from build123d import *

# Parameters (mm, degrees)
F0_W     = 20.1
F0_H     = 40.9
F0_W_2   = 15.1
F0_H_2   = 35.9
F1_DEPTH = 22
F2_DEPTH = 19.5
F4_R     = 1.695
F5_DEPTH = 25
F7_W     = 3.375
F7_H     = 4.11
F8_DEPTH = 25


with BuildPart() as f1:
    # F0 (on Top) → F1 (new body)
    with BuildSketch(Plane.XY):
        with Locations((7.55, 24.2)):
            Rectangle(F0_W, F0_H)
        with Locations((7.55, 24.2)):
            Rectangle(F0_W_2, F0_H_2, mode=Mode.SUBTRACT)
        with Locations((7.55, 24.2)):
            Rectangle(F0_W_2, F0_H_2)
    extrude(amount=F1_DEPTH)

    # F0 (on Top) → F2 (cut)
    with BuildSketch(Plane.XY):
        with Locations((7.55, 24.2)):
            Rectangle(F0_W_2, F0_H_2)
    extrude(amount=F2_DEPTH, mode=Mode.SUBTRACT)

    # F4 (on offset) → F5 (cut)
    with BuildSketch(Plane.XY.offset(22)):
        with Locations((4.5, 37.65)):
            Circle(F4_R)
        with Locations((10.6, 37.65)):
            Circle(F4_R)
        with Locations((4.5, 10.75)):
            Circle(F4_R)
        with Locations((10.6, 10.75)):
            Circle(F4_R)
    extrude(amount=-F5_DEPTH, mode=Mode.SUBTRACT)

    # F7 (on offset) → F8 (cut)
    with BuildSketch(Plane(origin=(0, 44.65, 0), x_dir=(-1, 0, 0), z_dir=(0, 1, 0))):
        with Locations((-5.8625, 15.2)):
            Rectangle(F7_W, F7_H)
        with Locations((-9.2375, 15.2)):
            Rectangle(F7_W, F7_H)
    extrude(amount=-F8_DEPTH, mode=Mode.SUBTRACT)


solid = f1.part
Part model, mm, in its own coordinate system. A direction names the side the tool comes from. Coordinates: 2 decimals unless noted, no trailing zeros. Loops run counter-clockwise (first coordinate to the right, second up) from the corner with the lowest first, then second, coordinate; pieces in that order, holes last. Notation, with made-up numbers: M 12.5,25.25 L 27.5,25.25 A17 cw 27.5,54.25 Z; hole C 39.25,29.5 d3. An arc over 180 degrees is marked long. Use a Markdown table: item, result. Add a question column.
Q1. Which spindle directions (+Z, -Z, +X, -X, +Y, -Y) get a long thin tool onto all of the face, cutting with end or side? Do faces 5 (the flat face through (15.1, 24, 10)), 6 (the flat face through (8, 43, 17.255)), 7 (the flat face through (-1, 23, 0)). Say none if no direction does.
Q2. Cut at A-A (y = 10.75). Write the cut outline in (x, z) (3 decimals), and give its area (3 significant figures).
Q3. Pin check, flat tips, straight feed: P1, Ø4, axis at x = 13, y = 25.5, coming from the -Z side; P2, Ø4, axis at x = 10.6, y = 10.75, coming from the +Z side. Stop position of each tip, or through.
Q4. Mould opens along Z. For faces 1 (the flat face through (8, 43, 13.145)), 2 (the flat face through (7, 24, 22)), 3 (the flat face through (4.175, 43, 15)), 4 (the flat face through (17.6, 24, 11)) say: +Z half, -Z half, draft (parallel to the pull), parting line (faces both ways), or undercut.
Q5. Probe L1, parallel to Y at x = 4.5, z = 20.7 (3 decimals); L2, parallel to X at y = 13, z = 4; L3, parallel to Y at x = 5.75, z = 11.5. List the from-to ranges inside material, lowest first.
Q6. Cut at B-B (z = 18.25). Write the cut outline in (x, y).
Q7. Cut at D-D (x = 0.75). Write the cut outline in (y, z).
Q8. Cut at C-C (y = 21). Write the cut outline in (x, z).
Worked out:
| question | item | result |
|---|---|---|
| 1 | face 5 | -Z |
| 1 | face 6 | +Y |
| 1 | face 7 | -Z, +X, -X, +Y, -Y |
| 2 | outline | M -2.5,0 L 0,0 L 0,19.5 L 2.805,19.5 L 2.805,22 L -2.5,22 Z; M 6.195,19.5 L 8.905,19.5 L 8.905,22 L 6.195,22 Z; M 12.295,19.5 L 15.1,19.5 L 15.1,0 L 17.6,0 L 17.6,22 L 12.295,22 Z |
| 2 | area | 131 mm2 |
| 3 | P1 | stops at z = 19.5 |
| 3 | P2 | stops at z = 22 |
| 4 | face 1 | undercut |
| 4 | face 2 | +Z half |
| 4 | face 3 | undercut |
| 4 | face 4 | draft |
| 5 | L1 | y = 3.75 to 9.055, 12.445 to 35.955, 39.345 to 44.65 |
| 5 | L2 | x = -2.5 to 0, 15.1 to 17.6 |
| 5 | L3 | y = 3.75 to 6.25, 42.15 to 44.65 |
| 6 | outline | M -2.5,3.75 L 17.6,3.75 L 17.6,44.65 L -2.5,44.65 Z; hole M 0,6.25 L 15.1,6.25 L 15.1,42.15 L 0,42.15 Z |
| 7 | outline | M 3.75,0 L 6.25,0 L 6.25,19.5 L 42.15,19.5 L 42.15,0 L 44.65,0 L 44.65,22 L 3.75,22 Z |
| 8 | outline | M -2.5,0 L 0,0 L 0,19.5 L 15.1,19.5 L 15.1,0 L 17.6,0 L 17.6,22 L -2.5,22 Z |
